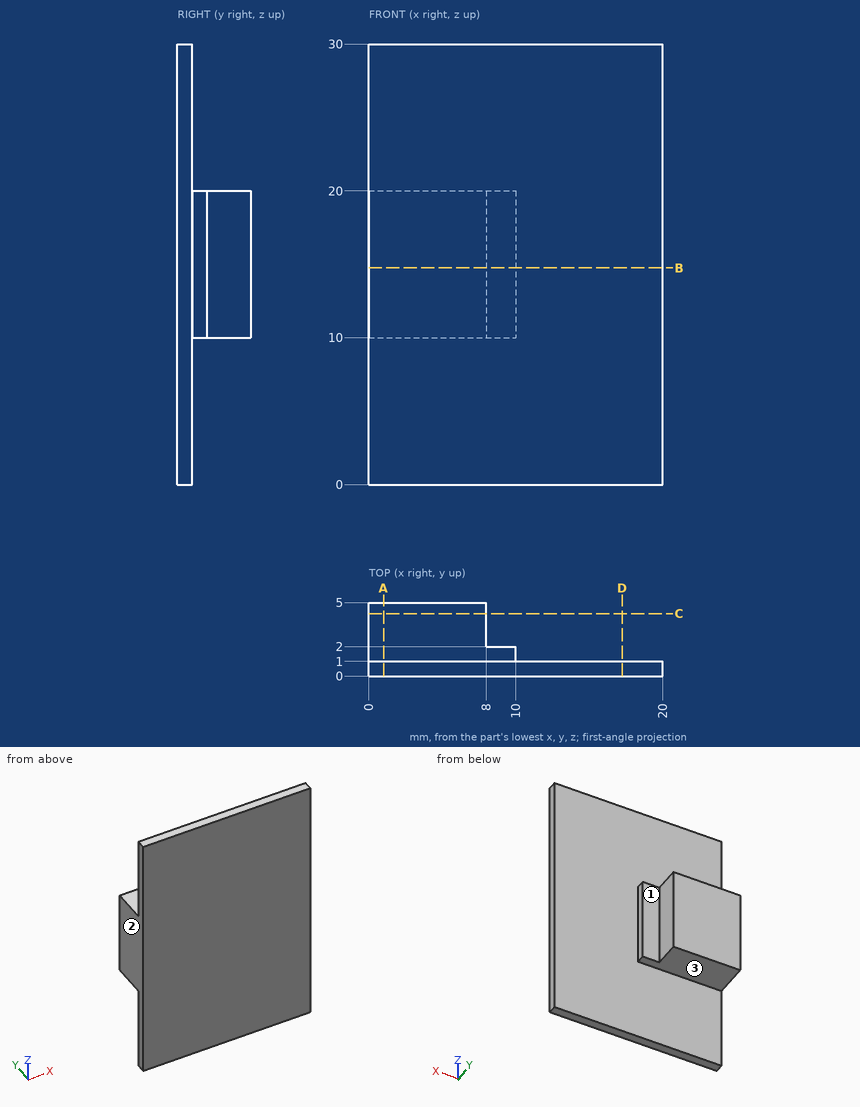
Drawing for the job (mm, zero at the part's lowest x, y, z). A direction names the side the tool comes from. Coordinates: 2 decimals unless noted, no trailing zeros. Order: outer loops, then holes, each group sorted by start corner. A loop starts at its lowest first (then second) coordinate and runs counter-clockwise, first axis right, second up. Notation, with made-up numbers: (-11, -5.75) - (5, -5.75) arc R25 cw to (5, 32.25) - close; hole circle Ø9 at (-35.75, -16). An arc over 180 degrees is marked (long way). Use a Markdown table: item, result. Add a question column.
(1) Saw through at A-A (x = 1). Give the cut face in (y, z).
(2) Drill centre lines: line 1 along Y through (x, z) = (3.75, 8.75); line 2 along Z through (x, y) = (2.25, 2.1); line 3 along X through (y, z) = (1.7, 17.25). Where is each one in solid material? Low to high. Write a range as [from, to].
(3) Which spindle directions (+Z, -Z, +X, -X, +Y, -Y) get a long thin tool onto all of the face, cutting with end or side? Do the marked faces 1, 2 and 3. Say none if no direction does.
(4) Flat gauge pins, fed straight in: pin 1 (3 mm diameter, centred on y = 4.5, z = 13, fed in from -X); pin 2 (1.6 mm diameter, centred on x = 9.5, z = 16, fed in from +Y); pin 3 (0.9 mm diameter, centred on y = 3.5, z = 16.5, fed in from +X); pin 4 (2 mm diameter, centred on x = 11, y = 3.5, fed in from -Z). Where does each tip first touch, or does it go through?
(5) Saw through at D-D (x = 17.25). Give the cut face in (y, z), then the cut area to 3 significant figures.
(6) Saw through at B-B (z = 14.75). Give the cut face in (x, y).
(7) Saw through at C-C (y = 4.25). Give the cut face in (x, z), then the cut area to 3 significant figures.
Solved:
| question | item | result |
|---|---|---|
| 1 | outline | (0, 0) - (1, 0) - (1, 10) - (5, 10) - (5, 20) - (1, 20) - (1, 30) - (0, 30) - close |
| 2 | line 1 | y = [0, 1] |
| 2 | line 2 | z = [10, 20] |
| 2 | line 3 | x = [0, 10] |
| 3 | face 1 | +Z, -Z, +X, +Y |
| 3 | face 2 | +Z, -Z, -X, +Y, -Y |
| 3 | face 3 | -Z, +X, -X, +Y |
| 4 | pin 1 | stops at x = 0 |
| 4 | pin 2 | stops at y = 2 |
| 4 | pin 3 | stops at x = 8 |
| 4 | pin 4 | passes through |
| 5 | outline | (0, 0) - (1, 0) - (1, 30) - (0, 30) - close |
| 5 | area | 30.0 mm² |
| 6 | outline | (0, 0) - (20, 0) - (20, 1) - (10, 1) - (10, 2) - (8, 2) - (8, 5) - (0, 5) - close |
| 7 | outline | (0, 10) - (8, 10) - (8, 20) - (0, 20) - close |
| 7 | area | 80.0 mm² |
